```python
from build123d import *

# Parameters (mm, degrees)
SKETCH_W       = 12
SKETCH_H       = 17.5
PAD_DEPTH      = 1.5
PAD_DEPTH_BACK = 10
SKETCH001_R    = 0.9
PAD001_DEPTH   = 10
PAD002_DEPTH   = 5
FILLET_R       = 1
FILLET001_R    = 1
FILLET002_R    = 1
SKETCH003_W    = 5.5
SKETCH003_H    = 7
PAD003_DEPTH   = 1.8
SKETCH004_R    = 2
PAD004_DEPTH   = 0.5
SKETCH005_R    = 2
PAD005_DEPTH   = 7
PAD005_TAPER   = -60


with BuildPart() as part:
    # Sketch → Pad (new body, two sides)
    with BuildSketch(Plane.XY) as pad_sk:
        Rectangle(SKETCH_W, SKETCH_H)
    extrude(amount=PAD_DEPTH)
    extrude(pad_sk.sketch, amount=-PAD_DEPTH_BACK)

    # Sketch001 → Pad001 (join)
    with BuildSketch(Plane.XY):
        with Locations((-3.25, 6)):
            Circle(SKETCH001_R)
        with Locations((-3.25, -6)):
            Circle(SKETCH001_R)
    extrude(amount=PAD001_DEPTH)

    # Sketch002 → Pad002 (join, symmetric)
    with BuildSketch(Plane.XZ):
        with BuildLine():
            ThreePointArc((13.745967, -10), (12.324555, -3.101021), (6, 0))
            Line((6, -10), (6, 0))
            Line((13.745967, -10), (6, -10))
        make_face()
    extrude(amount=PAD002_DEPTH, both=True)

    # Fillet
    fillet_edges = [part.edges().sort_by_distance(p)[0] for p in [
        (6, -8.75, -4.25),
        (-6, -8.75, -4.25),
        (6, 8.75, -4.25),
        (-6, 8.75, -4.25),
    ]]
    fillet(fillet_edges, radius=FILLET_R)

    # Fillet001
    fillet001_edges = [part.edges().sort_by_distance(p)[0] for p in [
        (12.324555, -5, -3.101021),
        (12.324555, 5, -3.101021),
    ]]
    fillet(fillet001_edges, radius=FILLET001_R)

    # Fillet002
    fillet002_edges = [part.edges().sort_by_distance(p)[0] for p in [
        (6, -5, -5.5),
    ]]
    fillet(fillet002_edges, radius=FILLET002_R)

    # Sketch003 (on Face6 of Fillet002) → Pad003 (join)
    with BuildSketch(Plane.XY.offset(1.5)):
        with Locations((-3.25, 0)):
            Rectangle(SKETCH003_W, SKETCH003_H)
    extrude(amount=PAD003_DEPTH)

    # Sketch004 (on Face28 of Pad003) → Pad004 (join)
    with BuildSketch(Plane.XY.offset(3.3)):
        with Locations((-3.25, -0.25)):
            Circle(SKETCH004_R)
    extrude(amount=PAD004_DEPTH)

    # Sketch005 (on Face32 of Pad004) → Pad005 (join)
    with BuildSketch(Plane.XY.offset(3.8)):
        with Locations((-3.25, -0.25)):
            Circle(SKETCH005_R)
    extrude(amount=PAD005_DEPTH, taper=PAD005_TAPER)


solid = part.part
```
Work out the finished part from the listing and answer in its coordinate system (mm). A direction names the side the tool comes from. Round coordinates to 2 decimals unless told otherwise and drop trailing zeros. Loops run counter-clockwise (first coordinate to the right, second up) from the corner with the lowest first, then second, coordinate; pieces in that order, holes last. Notation, with made-up numbers: M 75.25,58 L 79.25,58 A20 cw 79.25,66 Z; hole C 86,53 d1. An arc over 180 degrees is marked long. Use CSV: the item, a comma, the result in double quotes.
Q1. Consider L1, parallel to Y at x = -4, z = 5.25; L2, parallel to Z at x = 3, y = -4.5; L3, parallel to Z at x = -2, y = 4.5. Determine where each line is inside the solid, lowest interval first.
Determined:
L1,"-6.5 to -5.5, -4.7 to 4.2, 5.5 to 6.5"
L2,"-10 to 1.5, 7.01 to 10.8"
L3,"-10 to 1.5, 5.48 to 10.8"
Q2. A tool of negligible diameter and unlimited length cuts with its end or side. For faces 1 (the cylindrical face through (-3.7, -2.2, 3.5)), 2 (the cylindrical face through (-5.715, -8.449, -4.17)), 3 (the cylindrical face through (-5.715, 8.449, -4.33)), from which of +Z, -Z, +X, -X, +Y, -Y can it reach the whole face along a straight path? Write none if from no direction.
Determined:
face 1,"none"
face 2,"-Z, -X, -Y"
face 3,"-Z, -X, +Y"
Q3. Each of these flat-tipped pins is pushed along its axis until it touches: pin 1 (8 mm diameter, centred on y = -2.5, z = -5.5, fed in from -X); pin 2 (8 mm diameter, centred on x = -0.5, z = -7, fed in from -Y); pin 3 (0.9 mm diameter, centred on x = -3, z = 2.5, fed in from +Y); pin 4 (1 mm diameter, centred on x = 5.5, z = 6, fed in from +Y). Where does it stop, or does it pass through?
Determined:
pin 1,"x = -6"
pin 2,"y = -8.75"
pin 3,"y = 6.9"
pin 4,"through"
Q4. The mould has two halves that part along Y. Classify faces 4 (the flat face through (-2, 2, 3.3)), 5 (the cylindrical face through (6.285, -5.301, -5.473)), 6 (the cylindrical face through (6.248, 0.056, 0.285)), 7 (the cylindrical face through (-3.445, -6.879, 3.957)): pulls with the +Y half, pulls with the -Y half, needs draft (parallel to the pull), parting line crosses it, or undercut.
Determined:
face 4,"undercut"
face 5,"pulls with the -Y half"
face 6,"needs draft"
face 7,"undercut"
Q5. Section A-A, the plane z = 2.25 is taken. Determine the outline of the cut face in (x, y).
Determined:
outline,"M -6,-3.5 L -0.5,-3.5 L -0.5,3.5 L -6,3.5 Z; C -3.25,-6 d1.8; C -3.25,6 d1.8"
